Work out the finished part from the listing and answer in its coordinate system (mm). A direction names the side the tool comes from. Round coordinates to 2 decimals unless told otherwise and drop trailing zeros. Order: outer loops, then holes, each group sorted by start corner. A loop starts at its lowest first (then second) coordinate and runs counter-clockwise, first axis right, second up. Notation, with made-up numbers: (21.5, 49.5) -> (37.5, 49.5) arc R34 cw to (37.5, 85.5) -> close; hole circle Ø9 at (58, 51.25). An arc over 180 degrees is marked (long way). Use one line per item in the form item = value.
Autodesk Inventor part; units mm, degrees
ref_plane "YZ Plane" through (0, 0, 0) normal (1, 0, 0) x (0, 1, 0)
ref_plane "XZ Plane" through (0, 0, 0) normal (0, 1, 0) x (-1, 0, 0)
ref_plane "XY Plane" through (0, 0, 0) normal (0, 0, 1) x (1, 0, 0)
sketch "Sketch1" plane through (0, 0, 0) normal (0, 0, 1) x (1, 0, 0)
  line L0 (-6.9, 7.5) -> (6.9, 7.5)
  line L1 (6.9, 7.5) -> (6.9, -7.5)
  line L2 (6.9, -7.5) -> (-6.9, -7.5)
  line L3 (-6.9, -7.5) -> (-6.9, 7.5)
  line L4 (0, -10.5) -> (0, 10.5)
  line L5 (-9.66, 0) -> (9.66, 0)
  point P0 (0, 0)
  dimension "d0" = 13.8
  dimension "d9" = 15
extrude "Extrusion1" add sketch "Sketch1" along normal blind 2.5
sketch "Sketch3" plane through (0, 0, 2.5) normal (0, 0, 1) x (1, 0, 0)
  line L0 (6.9, 7.5) -> (-6.9, 7.5)
  line L1 (-6.9, -7.5) -> (6.9, -7.5)
  line L2 (-6.9, 7.5) -> (-5.4, 7.5)
  line L3 (-5.4, 7.5) -> (-5.4, -7.5)
  line L4 (-5.4, -7.5) -> (-6.9, -7.5)
  line L5 (-6.9, -7.5) -> (-6.9, 7.5)
  line L6 (6.9, -7.5) -> (6.9, 7.5)
  line L7 (6.9, 7.5) -> (5.4, 7.5)
  line L8 (5.4, 7.5) -> (5.4, -7.5)
  line L9 (5.4, -7.5) -> (6.9, -7.5)
  line L10 (6.9, -7.5) -> (6.9, 7.5)
  point P0 (0, 0)
  point P1 (5.4, 7.5)
  point P2 (5.4, -7.5)
  dimension "d11" = 1.5
  dimension "d12" = 1.5
extrude "Extrusion3" add sketch "Sketch3" along normal blind 2 contours L6 L1 L8 L0 | L3 L1 L5 L0
fillet "Fillet2" radius 2 2 edges at (-5.4, 0, 2.5) (5.4, 0, 2.5)
fillet "Fillet2" radius 0.4 6 edges at (-5.4, 0, 4.5) (-6.9, 0, 4.5) (5.4, 0, 4.5) (6.9, 0, 4.5) (6.9, 0, 0) (-6.9, 0, 0)
sketch "Sketch4" plane through (0, 0, 2.5) normal (0, 0, 1) x (1, 0, 0)
  line L0 (-3.4, -7.5) -> (3.4, -7.5)
  arc A0 (-3, -7.5) -> (3, -7.5) centre (0, -7.5) ccw
  point P0 (0, 0)
  dimension "d17" = 3
extrude "Extrusion4" add sketch "Sketch4" against normal up to surface (2.5 mm away)
sketch "Sketch5" plane through (0, 0, 0) normal (0, 0, -1) x (-1, 0, 0)
  circle A0 centre (0, -0.5) radius 3.25
  line L0 (-3, -7.5) -> (-6.5, -7.5) construction
  line L1 (0, -15.3299) -> (0, 11.305)
  arc A1 (-3, -7.5) -> (3, -7.5) centre (0, -7.5) ccw
  point P0 (0, 0)
  dimension "d20" = 6.5
  dimension "d21" = 7
extrude "Extrusion5" cut sketch "Sketch5" against normal blind 1
chamfer "Chamfer2" distance 0.2 angle 45 16 edges at (0, -10.5, 2.5) (0, -10.5, 0) (-4.75, -7.5, 0) (6.7828, -7.5, 4.3828) (-6.7828, -7.5, 0.1172) (6.9, -7.5, 2.25) (6.1332, -7.5, 4.5) (-6.1332, -7.5, 4.5) (5.5082, -7.5, 4.4055) (-5.5082, -7.5, 4.4055) (-6.7828, -7.5, 4.3828) (4.6911, -7.5, 2.9725) (-4.6911, -7.5, 2.9725) (-3.2001, -7.5, 2.5) (3.2001, -7.5, 2.5) (-6.9, -7.5, 2.25)
chamfer "Chamfer3" distance 1 angle 30 1 edges at (3.25, -0.5, 0) measured on face at (-3.2395, -0.7615, 0.6667)
properties part number "Test_SampleHolder_Plate_M8Screw_big"
Item 1: Determine the mould class of faces 4 (the flat face through (5, -7.5, 2)), 5 (the cylindrical face through (-4.71, 0, 2.99)), 6 (the flat face through (0, 0, 1)) for opening direction Y: released by +Y, released by -Y, zero draft, split by the parting line, or undercut.
Findings:
face_4 = released by -Y
face_5 = zero draft
face_6 = undercut
Item 2: The part is cut by section B-B, the plane z = 1.8. Give the vertices of the cut face in (x, y), and give its area (3 significant figures).
Findings:
outline = (-6.9, -7.3) -> (-6.7, -7.5) -> (-3, -7.5) arc R3 ccw to (3, -7.5) -> (6.7, -7.5) -> (6.9, -7.3) -> (6.9, 7.5) -> (-6.9, 7.5) -> close
area = 221 mm^2
Item 3: Consider line 1 along Z through (x, y) = (1.25, 0.5); line 2 along Y through (x, z) = (6.25, 0.3); line 3 along X through (y, z) = (-2, 2.85). Determine where each line is inside the solid, lowest interval first.
Findings:
line_1 = 1 to 2.5
line_2 = -7.5 to 7.5
line_3 = -6.9 to -4.53, 4.53 to 6.9
Item 4: Flat-ended cylindrical pins translate along their axes: P1, Ø2, axis at x = 1.5, y = 1, coming from the -Z side; P2, Ø1.9, axis at x = 5, z = 3, coming from the -Y side; P3, Ø4, axis at x = 0, y = 1, coming from the -Z side. Find the tip coordinate at first contact, or state that the pin passes through.
Findings:
P1 = 1
P2 = -7.5
P3 = 0.57
Item 5: For faces 1 (the flat face through (0, 7.5, 2)), 2 (the cylindrical face through (4.676, -0.004, 2.96)), 3 (the flat face through (-5, -7.5, 2)), determine the directions among +Z, -Z, +X, -X, +Y, -Y from which every point of the face is accessible in a straight line to the end or side of a thin tool.
Findings:
face_1 = +Z, -Z, +X, -X, +Y
face_2 = +Z, +Y, -Y
face_3 = +Z, -Z, -X, -Y
